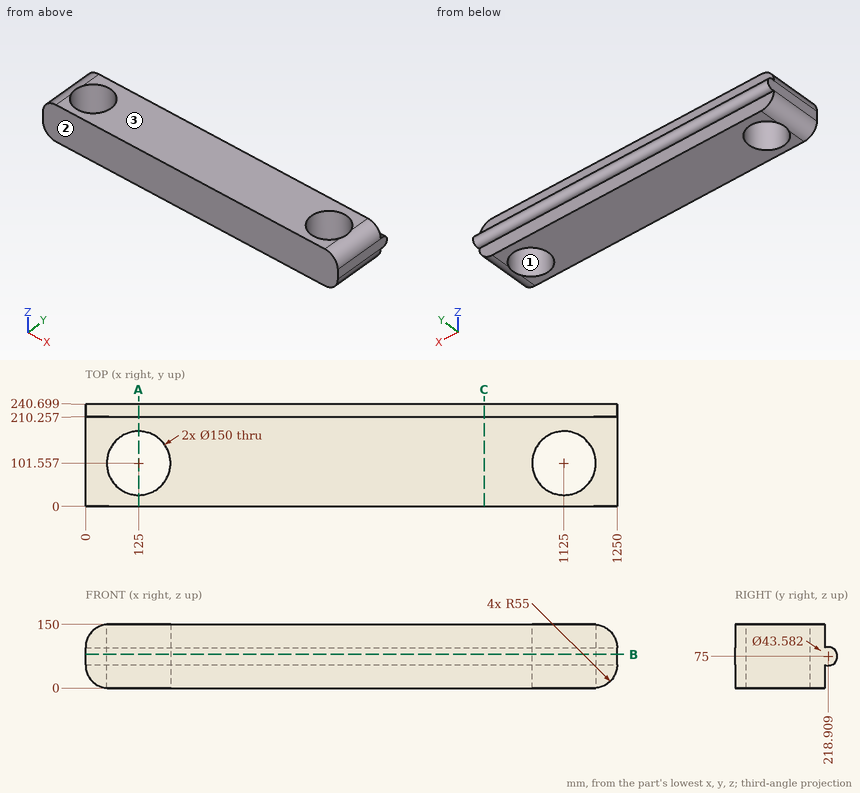
Part print with two shaded views. Sizes in mm from the minimum x, y, z corner. Coordinates: 2 decimals unless noted, no trailing zeros. Order: outer loops, then holes, each group sorted by start corner. A loop starts at its lowest first (then second) coordinate and runs counter-clockwise, first axis right, second up.
(1) Saw through at B-B, the plane z = 79.5. Write the cut outline in (x, y).
Solution:
outline: (0, 0) - (1250, 0) - (1250, 240.23) - (0, 240.23) - close; hole circle Ø150 at (125, 101.56); hole circle Ø150 at (1125, 101.56)
(2) Mould opens along Y. For the marked faces 1, 2 and 3 say: released by +Y, released by -Y, zero draft, split by the parting line, or undercut.
Solution:
face 1: undercut
face 2: released by -Y
face 3: zero draft
(3) Pin check, flat tips, straight feed: pin 1 Ø10 at (y, z) = (103.5, 109) entering from +X; pin 2 Ø6 at (x, z) = (608, 44) entering from +Y; pin 3 Ø10 at (y, z) = (65.5, 17) entering from +X. Stop position of each tip, or through.
Solution:
pin 1: stops at x = 1249.26
pin 2: stops at y = 210.26
pin 3: stops at x = 1239
(4) Saw through at A-A, the plane x = 125. Write the cut outline in (y, z).
Solution:
outline: (0, 0) - (26.56, 0) - (26.56, 150) - (0, 150) - close; (176.56, 0) - (210.26, 0) - (210.26, 55) arc R21.79 ccw (long way) to (210.26, 95) - (210.26, 150) - (176.56, 150) - close
(5) Drill centre lines: L1, parallel to X at y = 76.5, z = 125.5; L2, parallel to X at y = 62.5, z = 29 (1 decimal); L3, parallel to Y at x = 1127, z = 124. Where is each one in solid material? Low to high.
Solution:
L1: x = 9.23 to 54.31, 195.69 to 1054.31, 1195.69 to 1240.77
L2: x = 6.5 to 61, 189 to 1061, 1189 to 1243.5
L3: y = 0 to 26.58, 176.53 to 210.26
(6) Saw through at C-C, the plane x = 937.5. Write the cut outline in (y, z).
Solution:
outline: (0, 0) - (210.26, 0) - (210.26, 55) arc R21.79 ccw (long way) to (210.26, 95) - (210.26, 150) - (0, 150) - close
